Here's how the part is built. I have some questions about the finished solid (model axes, mm). A direction names the side the tool comes from. Round coordinates to 2 decimals unless told otherwise and drop trailing zeros. Write each loop counter-clockwise with the first axis right and the second up, starting at its lowest first coordinate (ties: lowest second). Pieces come first, ordered by that corner, then holes. Notation, with made-up numbers: (28.5, -27) -> (53.5, -27) arc R11 cw to (53.5, -21) -> close; hole circle Ø6 at (17, 25). An arc over 180 degrees is marked (long way). Answer as CSV lines item,"result".
from build123d import *

# Parameters (mm, degrees)
BOSS_EXTRUDE1_DEPTH = 3.175


with BuildPart() as part:
    # Sketch1 → Boss-Extrude1 (new body)
    with BuildSketch(Plane.XY):
        with BuildLine():
            Line((-38.1, 31.27375), (-38.1, 57.785))
            Line((-38.1, 57.785), (-42.216961876, 57.167455719))
            ThreePointArc((-42.216961876, 57.167455719), (-46.086650336, 55.031442621), (-47.625, 50.887709878))
            Line((-47.625, 50.887709878), (-47.625, 6.35))
            ThreePointArc((-47.625, 6.35), (-45.765128061, 1.859871939), (-41.275, 0))
            Line((-41.275, 0), (-38.1, 0))
            Line((-38.1, 0), (-38.1, 26.51125))
            ThreePointArc((-38.1, 26.51125), (-40.48125, 28.8925), (-38.1, 31.27375))
        make_face()
        with BuildLine():
            Line((0, 41.275), (0, 56.126459878))
            ThreePointArc((0, 56.126459878), (-2.206267257, 60.938110214), (-7.291961876, 62.406205719))
            Line((-7.291961876, 62.406205719), (-38.1, 57.785))
            Line((-38.1, 57.785), (-38.1, 31.27375))
            ThreePointArc((-38.1, 31.27375), (-36.416201977, 30.576298023), (-35.71875, 28.8925))
            ThreePointArc((-35.71875, 28.8925), (-36.416201977, 27.208701977), (-38.1, 26.51125))
            Line((-38.1, 26.51125), (-38.1, 0))
            Line((-38.1, 0), (-26.9875, 0))
            Line((-26.9875, 0), (-26.9875, 3.175))
            Line((-26.9875, 3.175), (-14.2875, 3.175))
            Line((-14.2875, 3.175), (-14.2875, 0))
            Line((-14.2875, 0), (-6.35, 0))
            ThreePointArc((-6.35, 0), (-1.859871939, 1.859871939), (0, 6.35))
            Line((0, 6.35), (0, 22.225))
            Line((0, 22.225), (-3.175, 22.225))
            Line((-3.175, 22.225), (-3.175, 41.275))
            Line((-3.175, 41.275), (0, 41.275))
        make_face()
    extrude(amount=BOSS_EXTRUDE1_DEPTH)


solid = part.part
Item 1: Suppose I cut it at B-B, the plane y = 39.5. List the corners of the cut face in (x, z) for me (3 decimals).
Results found:
outline,"(-47.625, 0) -> (-3.175, 0) -> (-3.175, 3.175) -> (-47.625, 3.175) -> close"
Item 2: I need wall thicknesses on L1, parallel to X at y = 29, z = 1.2 (3 decimals); L2, parallel to Y at x = -36, z = 1.3; L3, parallel to Y at x = -6.5, z = 2.2. Which ranges of each line are inside material? Lowest first, please.
Results found:
L1,"x = -47.625 to -40.479, -35.721 to -3.175"
L2,"y = 0 to 27.77, 30.02 to 58.1"
L3,"y = 0 to 62.47"
Item 3: Will these pins go through, and if not, where does the flat tip stop? pin 1 (1 mm diameter, centred on y = 1.5, z = 1.5, fed in from -X); pin 2 (1.6 mm diameter, centred on x = -22, z = 1, fed in from -Y) (3 decimals); pin 3 (1.6 mm diameter, centred on y = 33.5, z = 1.5, fed in from +X) (3 decimals).
Results found:
pin 1,"stops at x = -45.9"
pin 2,"stops at y = 3.175"
pin 3,"stops at x = -3.175"
Item 4: Suppose I cut it at C-C, the plane x = -17. List the corners of the cut face in (y, z) for me (3 decimals).
Results found:
outline,"(3.175, 0) -> (60.95, 0) -> (60.95, 3.175) -> (3.175, 3.175) -> close"
Item 5: If we mould it in two halves opening along X, with no side actions, what happens to faces 4 (the flat face through (-10, 0, 2)), 5 (the flat face through (-14.288, 2, 2)), 6 (the cylindrical face through (-46.045, 55.079, 1.565))? For each: pulls with the +X half, pulls with the -X half, needs draft (parallel to the pull), parting line crosses it, or undercut.
Results found:
face 4,"needs draft"
face 5,"undercut"
face 6,"pulls with the -X half"
Item 6: For faces 1 (the flat face through (-24, 32, 3.175)), 2 (the flat face through (-21, 3.175, 2)), 3 (the flat face through (-3.175, 32, 2)), which set-ups out of +Z, -Z, +X, -X, +Y, -Y let a thin tool reach every point of the face, with its end or its side?
Results found:
face 1,"+Z, +X, -X, +Y, -Y"
face 2,"+Z, -Z, -Y"
face 3,"+Z, -Z, +X"
